Source: three-view drawing plus pictorial views. Frame: mm from the lowest corner of the part. A direction names the side the tool comes from. Give positions to 0.01 mm unless a question says otherwise; leave off trailing zeros. Write each loop counter-clockwise with the first axis right and the second up, starting at its lowest first coordinate (ties: lowest second). Pieces come first, ordered by that corner, then holes.
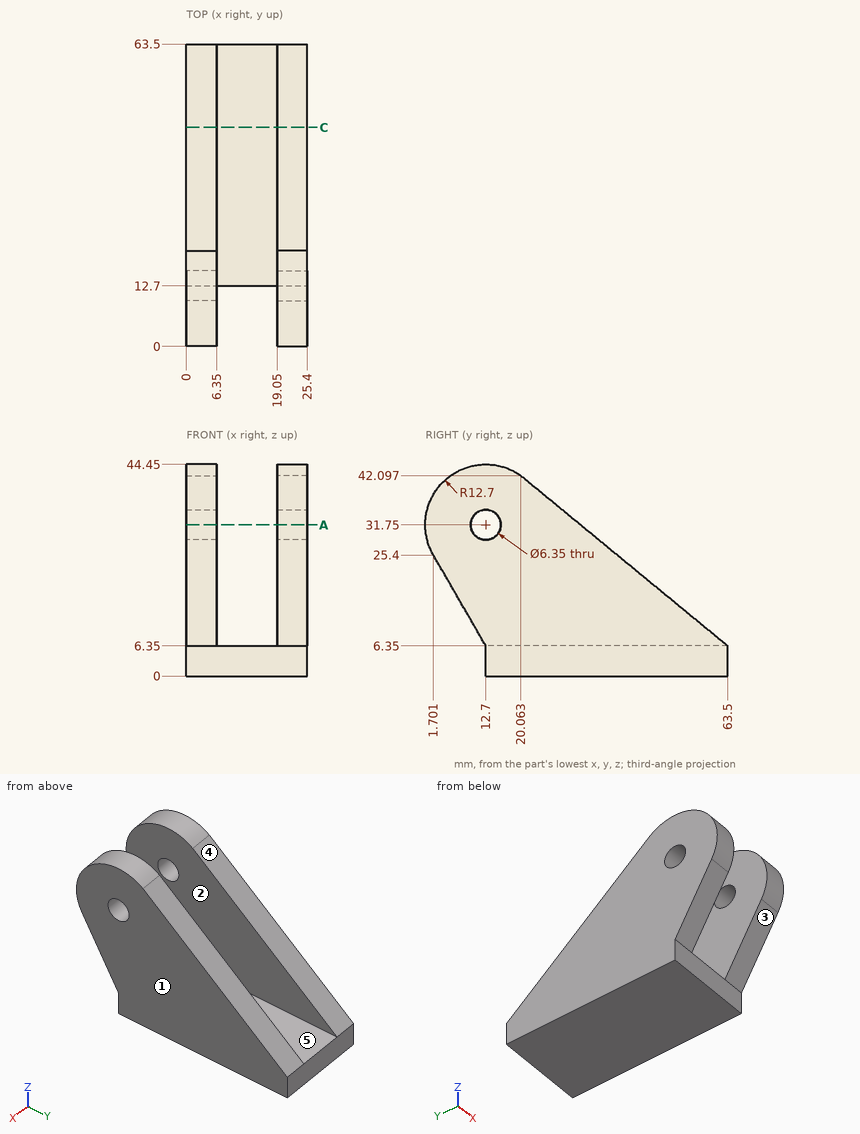
Q1. Section A-A on z = 31.75. Count the separate pieces of the cut face and the enclosed holes in it, plus the area to 3 significant figures.
Filled sheet:
separate pieces: 4
enclosed holes: 0
area: 334 mm2
Q2. Access query for the marked faces 4 and 5. Directions: +Z, -Z, +X, -X, +Y, -Y. A direction counts if a zero-diameter tool reaches every point of the face in a straight line with its end or side. Return the directions, or none.
Filled sheet:
face 4: +Z, +X, -X, +Y
face 5: +Z, +Y, -Y
Q3. Pin query (flat end, axial travel): P1, Ø1.9, axis at x = 18.5, z = 3, coming from the -Y side; P2, Ø4, axis at y = 12.7, z = 31.75, coming from the +X side; P3, Ø1, axis at x = 4, y = 18, coming from the +Z side; P4, Ø10, axis at x = 15, y = 48, coming from the +Z side. Return the tip coordinate at first contact, or that it passes through.
Filled sheet:
P1: stops at y = 12.7
P2: passes through
P3: stops at z = 43.51
P4: stops at z = 21.52
Q4. Section C-C on y = 46. Output: boundary loops of the cut face in (x, z), plus the area to 3 significant figures.
Filled sheet:
outline: (0, 0) - (25.4, 0) - (25.4, 20.75) - (19.05, 20.75) - (19.05, 6.35) - (6.35, 6.35) - (6.35, 20.75) - (0, 20.75) - close
area: 344 mm2
Q5. Ray query, line 1 along X through (y, z) = (19, 30.5); line 2 along Y through (x, z) = (21.75, 3); line 3 along Y through (x, z) = (22, 31.75) (1 decimal). Return the intervals inside material, ascending.
Filled sheet:
line 1: x = 0 to 6.35, 19.05 to 25.4
line 2: y = 12.7 to 63.5
line 3: y = 0 to 9.5, 15.9 to 32.6
Q6. Pull-direction query (X, two-part tool) for the marked faces 1, 2 and 3; classes: released by +X, released by -X, zero draft, split by the parting line, or undercut.
Filled sheet:
face 1: released by +X
face 2: undercut
face 3: zero draft
